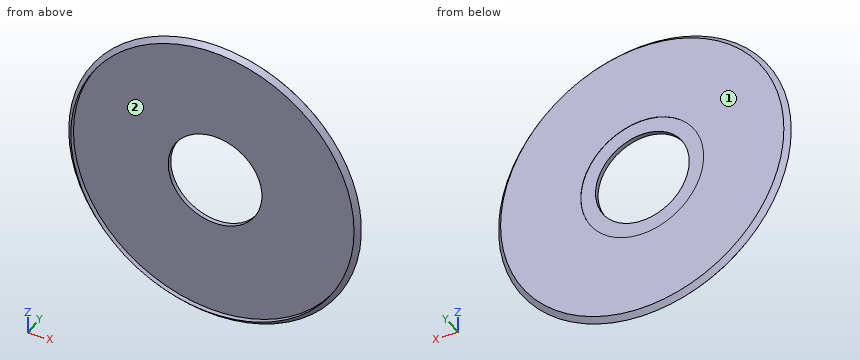
Autodesk Inventor part; units mm, degrees
ref_plane "YZ Plane" through (0, 0, 0) normal (1, 0, 0) x (0, 1, 0)
ref_plane "XZ Plane" through (0, 0, 0) normal (0, 1, 0) x (-1, 0, 0)
ref_plane "XY Plane" through (0, 0, 0) normal (0, 0, 1) x (1, 0, 0)
sketch "Sketch1" plane through (0, 0, 0) normal (0, 1, 0) x (-1, 0, 0)
  circle A0 centre (0, 0) radius 31.75
  circle A1 centre (0, 0) radius 10.16
  dimension "d0" = 63.5
  dimension "d1" = 20.32
extrude "Extrusion1" add sketch "Sketch1" along normal blind 2.032
sketch "Sketch2" plane through (0, 2.032, 0) normal (0, 1, 0) x (1, 0, 0)
  circle A0 centre (0, 0) radius 10.16
  circle A1 centre (0, 0) radius 31.75
  circle A2 centre (0, 0) radius 13.335
  dimension "d4" = 26.67
extrude "Extrusion2" cut sketch "Sketch2" against normal blind 0.06 contours A2
chamfer "Chamfer1" distance 1.016 angle 45 2 edges at (31.75, 2.032, 0) (31.75, 0, 0)
sketch "Sketch3" plane through (0, 0, 0) normal (0, -1, 0) x (1, 0, 0)
  circle A0 centre (0, 0) radius 10.16
  circle A1 centre (0, 0) radius 30.734
emboss "Emboss1" sketch "Sketch3" operation cut depth 1.016 direction (0, 1, 0)
properties part number "Si Frame Mk 3"
The model under review builds one solid part; all positions refer to its coordinate system, in mm. Face numbers are marked on the shaded views. Round coordinates to 2 decimals unless told otherwise and drop trailing zeros. Write each loop counter-clockwise with the first axis right and the second up, starting at its lowest first coordinate (ties: lowest second). Pieces come first, ordered by that corner, then holes. Notation, with made-up numbers: (8.25, 28.25) -> (27.25, 28.25) arc R28 ccw to (27.25, 54.25) -> close; hole circle Ø2 at (-21, -13). An arc over 180 degrees is marked (long way). Answer as a JSON object with one key per item and string values.
1. The part is to be moulded in two halves that separate along Z. For the marked faces 1 and 2, say which applies: pulls with the +Z half, pulls with the -Z half, needs draft (parallel to the pull), parting line crosses it, or undercut.
Results found:
{"face 1": "needs draft", "face 2": "undercut"}
2. Clearance check with a flat-ended pin moving along its axis: pin 1 (3 mm diameter, centred on x = -9.5, z = -1, fed in from -Y). State where the tip first meets the part, or that it passes through.
Results found:
{"pin 1": "stops at y = 1.02"}
3. To check wall thickness, follow line 1 along Y through (x, z) = (12, 15); line 2 along X through (y, z) = (0.95, -10); line 3 along Z through (x, y) = (10.5, 0.7). State the ranges of each line that lie inside material, in increasing order.
Results found:
{"line 1": "y = 1.02 to 2.03", "line 2": "x = -30.06 to -29.06, 29.06 to 30.06", "line 3": "z = -29.63 to -28.88, 28.88 to 29.63"}
4. We need section C-C on y = 0.4. State the section outline as (x, z) points, and give its area (3 significant figures).
Results found:
{"outline": "circle Ø62.27 at (0, 0); hole circle Ø61.47 at (0, 0)", "area": "77.7 mm^2"}
